```python
from build123d import *

# Parameters (mm, degrees)
SKETCH1_R           = 3
SKETCH1_R_2         = 6.375
BOSS_EXTRUDE1_DEPTH = 5.6
SKETCH2_R           = 6.375
CUT_EXTRUDE1_DEPTH  = 3.6
SKETCH3_R           = 4
CUT_EXTRUDE2_DEPTH  = 29.810093495


with BuildPart() as part:
    # Sketch1 → Boss-Extrude1 (new body)
    # profile 1 of 4: a face of its own
    with BuildSketch(Plane(origin=(0, 0, 0), x_dir=(1, 0, 0), z_dir=(0, 1, 0))):
        with BuildLine():
            ThreePointArc((-14.775889156, 1.860291889), (-17.90204805, -10.960217435), (-4.883341128, -13.116973989))
            ThreePointArc((-4.883341128, -13.116973989), (0, -11.447792844), (4.883341128, -13.116973989))
            ThreePointArc((4.883341128, -13.116973989), (17.993886057, -10.818294624), (14.477584826, 2.019381989))
            ThreePointArc((14.477584826, 2.019381989), (10.324072295, 5.960605919), (8.987628515, 11.52826525))
            ThreePointArc((8.987628515, 11.52826525), (0.169037816, 20.998412428), (-8.999004613, 11.866149428))
            ThreePointArc((-8.999004613, 11.866149428), (-10.506960828, 6.066196663), (-14.775889156, 1.860291889))
        make_face()
        with Locations(Location((0, 0, 0), (0, 0, 270))):
            Circle(SKETCH1_R, mode=Mode.SUBTRACT)
        with Locations((0, 12)):
            Circle(SKETCH1_R_2, mode=Mode.SUBTRACT)
        with Locations((10.392304845, -6)):
            Circle(SKETCH1_R_2, mode=Mode.SUBTRACT)
        with Locations((-10.392304845, -6)):
            Circle(SKETCH1_R_2, mode=Mode.SUBTRACT)
    # profile 2 of 4: a face of its own
    with BuildSketch(Plane(origin=(0, 0, 0), x_dir=(1, 0, 0), z_dir=(0, 1, 0))):
        with Locations((0, 12)):
            Circle(SKETCH1_R_2)
    # profile 3 of 4: a face of its own
    with BuildSketch(Plane(origin=(0, 0, 0), x_dir=(1, 0, 0), z_dir=(0, 1, 0))):
        with Locations((10.392304845, -6)):
            Circle(SKETCH1_R_2)
    # profile 4 of 4: a face of its own
    with BuildSketch(Plane(origin=(0, 0, 0), x_dir=(1, 0, 0), z_dir=(0, 1, 0))):
        with Locations((-10.392304845, -6)):
            Circle(SKETCH1_R_2)
    extrude(amount=BOSS_EXTRUDE1_DEPTH)

    # Sketch2 → Cut-Extrude1 (cut)
    with BuildSketch(Plane(origin=(0, 5.6, 0), x_dir=(1, 0, 0), z_dir=(0, 1, 0))):
        with Locations(Location((-10.392304845, -6, 0), (0, 0, 270))):
            Circle(SKETCH2_R)
        with Locations(Location((0, 12, 0), (0, 0, 270))):
            Circle(SKETCH2_R)
        with Locations(Location((10.392304845, -6, 0), (0, 0, 270))):
            Circle(SKETCH2_R)
    extrude(amount=-CUT_EXTRUDE1_DEPTH, mode=Mode.SUBTRACT)

    # Sketch3 → Cut-Extrude2 (cut, through all)
    with BuildSketch(Plane(origin=(0, 2, 0), x_dir=(1, 0, 0), z_dir=(0, 1, 0))):
        with Locations(Location((-10.392304845, -6, 0), (0, 0, 270))):
            Circle(SKETCH3_R)
        with Locations(Location((0, 12, 0), (0, 0, 270))):
            Circle(SKETCH3_R)
        with Locations(Location((10.392304845, -6, 0), (0, 0, 270))):
            Circle(SKETCH3_R)
    extrude(amount=-CUT_EXTRUDE2_DEPTH, mode=Mode.SUBTRACT)


solid = part.part
```
The model under review builds one solid part; all positions refer to its coordinate system, in mm. A direction names the side the tool comes from. Give positions to 0.01 mm unless a question says otherwise; leave off trailing zeros. Loops run counter-clockwise (first coordinate to the right, second up) from the corner with the lowest first, then second, coordinate; pieces in that order, holes last. Notation, with made-up numbers: (47, -21) -> (96, -21) arc R13 ccw to (96, -12) -> close; hole circle Ø4 at (32, -33.75). An arc over 180 degrees is marked (long way). Use CSV: the item, a comma, the result in double quotes.
1. Consider section C-C, the plane z = -8.5. Write out the cut boundary in (x, y), then the cut area to 3 significant figures.
Result:
outline,"(-9.46, 0) -> (-1.94, 0) -> (-1.94, 2) -> (-5.33, 2) -> (-5.33, 5.6) -> (-9.46, 5.6) -> close; (1.94, 0) -> (9.29, 0) -> (9.29, 5.6) -> (5.33, 5.6) -> (5.33, 2) -> (1.94, 2) -> close"
area,"58.9 mm²"
2. Consider section B-B, the plane z = 6. Write out the cut boundary in (x, y), then the cut area to 3 significant figures.
Result:
outline,"(-19.39, 0) -> (-14.39, 0) -> (-14.39, 2) -> (-16.77, 2) -> (-16.77, 5.6) -> (-19.39, 5.6) -> close; (-6.39, 0) -> (6.39, 0) -> (6.39, 2) -> (4.02, 2) -> (4.02, 5.6) -> (-4.02, 5.6) -> (-4.02, 2) -> (-6.39, 2) -> close; (14.39, 0) -> (19.39, 0) -> (19.39, 5.6) -> (16.77, 5.6) -> (16.77, 2) -> (14.39, 2) -> close"
area,"93.4 mm²"
3. Consider section A-A, the plane x = 0. Write out the cut boundary in (y, z) (3 decimals).
Result:
outline,"(0, -21) -> (5.6, -21) -> (5.6, -18.375) -> (2, -18.375) -> (2, -16) -> (0, -16) -> close; (0, -8) -> (2, -8) -> (2, -5.625) -> (5.6, -5.625) -> (5.6, -3) -> (0, -3) -> close; (0, 3) -> (5.6, 3) -> (5.6, 11.448) -> (0, 11.448) -> close"
4. The part is to be moulded in two halves that separate along Z. For faces 3 (the face through (-0.07, 2.76, 11.45)), 4 (the face through (-0.3, 0, -3.3)), 5 (the face through (3, 2, -9)), 6 (the face through (-2.44, 3.83, -6.11)), say which applies: +Z half, -Z half, draft (parallel to the pull), parting line (faces both ways), or undercut.
Result:
face 3,"+Z half"
face 4,"draft"
face 5,"undercut"
face 6,"undercut"
5. Consider section D-D, the plane x = -7. Write out the cut boundary in (y, z).
Result:
outline,"(0, -17.66) -> (5.6, -17.66) -> (5.6, 0.6) -> (2, 0.6) -> (2, 3.88) -> (0, 3.88) -> close; (0, 8.12) -> (2, 8.12) -> (2, 11.4) -> (5.6, 11.4) -> (5.6, 14.34) -> (0, 14.34) -> close"
6. To check wall thickness, follow probe 1 along X at (y, z) = (0.65, 6); probe 2 along X at (y, z) = (3.8, 6); probe 3 along X at (y, z) = (0.5, -12). State the ranges of each line that lie inside material, in increasing order. Write a range as from..to.
Result:
probe 1,"x = -19.39..-14.39, -6.39..6.39, 14.39..19.39"
probe 2,"x = -19.39..-16.77, -4.02..4.02, 16.77..19.39"
probe 3,"x = -9..-4, 4..9"
7. Machinability: for faces 1 (the face through (10.5, 2, 10.2)), 2 (the face through (-14.297, 1.014, 5.133)), which of the approach directions +Z, -Z, +X, -X, +Y, -Y give a long, thin tool a straight path to every point of the face, cutting with its end or side? Answer none if there is none.
Result:
face 1,"+Y"
face 2,"+Y, -Y"
8. For P1, Ø2, axis at y = 3.5, z = -12, coming from the +X side; P2, Ø1, axis at x = -9.5, z = 9.5, coming from the +Y side; P3, Ø1, axis at y = 1.5, z = -2.5, coming from the +X side, all flat-tipped, find the tip position at first contact; note any pin that passes through.
Result:
P1,"stops at x = 9"
P2,"stops at y = 2"
P3,"stops at x = 14.52"
